Answer from the drawing. Dimensions are ordinates in mm from the lowest x, y and z of the part. Coordinates: 2 decimals unless noted, no trailing zeros. Loops run counter-clockwise (first coordinate to the right, second up) from the corner with the lowest first, then second, coordinate; pieces in that order, holes last. Notation, with made-up numbers: (-10, 66.5) -> (2, 66.5) arc R25 cw to (2, 99.5) -> close; hole circle Ø6 at (37.25, 88.5). An arc over 180 degrees is marked (long way). Use a Markdown table: item, result.
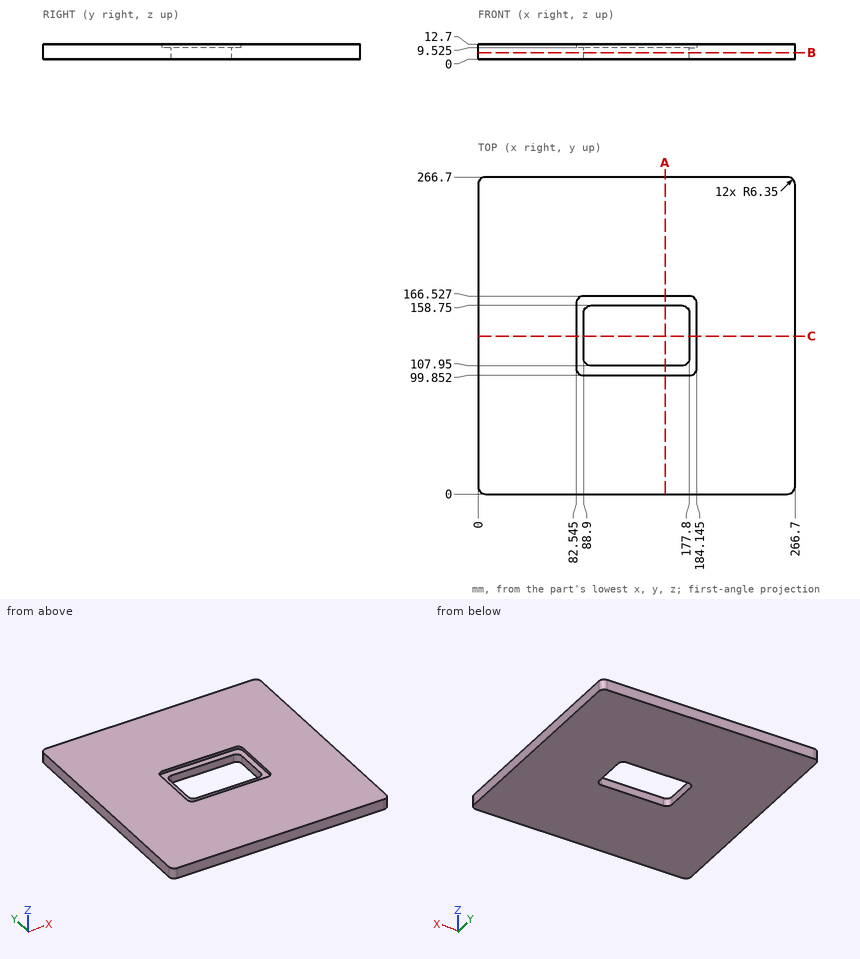
Q1. Consider line 1 (X direction, y = 135, z = 11.25) (3 decimals); line 2 (X direction, y = 116, z = 6); line 3 (Y direction, x = 113.5, z = 0.5). Determine where each line is inside the solid, lowest interval first. Write a range as [from, to].
Solved:
| item | result |
|---|---|
| line 1 | [0, 82.545], [184.145, 266.7] |
| line 2 | [0, 88.9], [177.8, 266.7] |
| line 3 | [0, 107.95], [158.75, 266.7] |
Q2. Section C-C on y = 133 is taken. Determine the outline of the cut face in (x, z) (3 decimals).
Solved:
| item | result |
|---|---|
| outline | (0, 0) -> (88.9, 0) -> (88.9, 9.525) -> (82.545, 9.525) -> (82.545, 12.7) -> (0, 12.7) -> close; (177.8, 0) -> (266.7, 0) -> (266.7, 12.7) -> (184.145, 12.7) -> (184.145, 9.525) -> (177.8, 9.525) -> close |
Q3. Section A-A on x = 157.5 is taken. Determine the outline of the cut face in (y, z) (3 decimals).
Solved:
| item | result |
|---|---|
| outline | (0, 0) -> (107.95, 0) -> (107.95, 9.525) -> (99.852, 9.525) -> (99.852, 12.7) -> (0, 12.7) -> close; (158.75, 0) -> (266.7, 0) -> (266.7, 12.7) -> (166.527, 12.7) -> (166.527, 9.525) -> (158.75, 9.525) -> close |
Q4. Given pin 1 Ø3 at (x, y) = (163.5, 66) entering from -Z, flat-ended and moving along its own axis, determine where the tip first touches the part or whether it passes through.
Solved:
| item | result |
|---|---|
| pin 1 | z = 0 |
Q5. Section B-B on z = 5.5 is taken. Determine the outline of the cut face in (x, y).
Solved:
| item | result |
|---|---|
| outline | (0, 6.35) arc R6.35 ccw to (6.35, 0) -> (260.35, 0) arc R6.35 ccw to (266.7, 6.35) -> (266.7, 260.35) arc R6.35 ccw to (260.35, 266.7) -> (6.35, 266.7) arc R6.35 ccw to (0, 260.35) -> close; hole (88.9, 114.3) arc R6.35 ccw to (95.25, 107.95) -> (171.45, 107.95) arc R6.35 ccw to (177.8, 114.3) -> (177.8, 152.4) arc R6.35 ccw to (171.45, 158.75) -> (95.25, 158.75) arc R6.35 ccw to (88.9, 152.4) -> close |
